from build123d import *

# Parameters (mm, degrees)
SKETCH1_R           = 3.555
SKETCH1_R_2         = 2.5
BOSS_EXTRUDE3_DEPTH = 6.35
BOSS_EXTRUDE4_START = -1.27
SKETCH1_5_R         = 3.555
SKETCH1_5_R_2       = 2.5
BOSS_EXTRUDE4_DEPTH = 1.27


with BuildPart() as part:
    # Sketch1 → Boss-Extrude3 (new body)
    # profile 1 of 2: a face of its own
    with BuildSketch(Plane.XY):
        Polygon((4.725, -2.271873309), (4.725, 2.271873309), (0.79, 4.543746619), (-3.145, 2.271873309), (-3.145, -2.271873309), (0.79, -4.543746619), align=None)
        with Locations((0.79, 0)):
            Circle(SKETCH1_R, mode=Mode.SUBTRACT)
    # profile 2 of 2: a face of its own
    with BuildSketch(Plane.XY):
        with Locations((0.79, 0)):
            Circle(SKETCH1_R)
        Circle(SKETCH1_R_2, mode=Mode.SUBTRACT)
    extrude(amount=BOSS_EXTRUDE3_DEPTH)

    # Sketch1_5 → Boss-Extrude4 (add)
    with BuildSketch(Plane.XY.offset(BOSS_EXTRUDE4_START)):
        with Locations((0.79, 0)):
            Circle(SKETCH1_5_R)
        Circle(SKETCH1_5_R_2, mode=Mode.SUBTRACT)
    extrude(amount=BOSS_EXTRUDE4_DEPTH)


solid = part.part
Here's how the part is built. I have some questions about the finished solid (model axes, mm). A direction names the side the tool comes from. Give positions to 0.01 mm unless a question says otherwise; leave off trailing zeros. Order: outer loops, then holes, each group sorted by start corner. A loop starts at its lowest first (then second) coordinate and runs counter-clockwise, first axis right, second up. Notation, with made-up numbers: M 14,81 L 51,81 A28 cw 51,111 Z; hole C -19,59 d10. An arc over 180 degrees is marked long. Answer as a JSON object with one key per item and string values. Group by question number.
1) Suppose I cut it at C-C, the plane y = 0. Write out the boundary of the cut face in (x, z) (3 decimals), plus the area to 3 significant figures.
2) We'd pull the mould along X, two halves only. Please class faces 3 (the cylindrical face through (-0.54, -2.44, 2.49)), 4 (the flat face through (3, 0, -1.27)), 5 (the cylindrical face through (4.18, 1.07, -0.64)), 6 (the flat face through (4.725, 0, 3)): pulls with the +X half, pulls with the -X half, needs draft (parallel to the pull), parting line crosses it, or undercut.
3) Suppose I cut it at B-B, the plane x = 0. Write out the boundary of the cut face in (y, z).
4) Suppose I cut it at D-D, the plane x = 3. Write out the boundary of the cut face in (y, z), plus the area to 3 significant figures.
5) I'm going to push a flat-ended pin straight in: pin 1 Ø4 at (x, z) = (4, 5) entering from -Y. Where does the tip first touch, or does it pass through?
6) Please list where these lines run through material, in increasing order: L1, parallel to Y at x = -0.75, z = 1; L2, parallel to Z at x = -2.75, y = 1.5; L3, parallel to Y at x = 0, z = 2.75. Write a range as [from, to].
7) Suppose I cut it at A-A, the plane z = 2.5. Write out the boundary of the cut face in (x, y) (3 decimals), plus the area to 3 significant figures.
8) On a 3-axis mill with a long thin cutter (end or side, diameter ignored), from which of +Z, -Z, +X, -X, +Y, -Y can I reach the whole of each face in a straight line? I mean faces 1 (the flat face through (1, -4, 0)), 2 (the flat face through (2.73, -3.424, 3.131)). Say none if no direction works.
Results found:
{
 "1": {"outline": "M -3.145,0 L -2.765,0 L -2.765,-1.27 L -2.5,-1.27 L -2.5,6.35 L -3.145,6.35 Z; M 2.5,-1.27 L 4.345,-1.27 L 4.345,0 L 4.725,0 L 4.725,6.35 L 2.5,6.35 Z", "area": "20.9 mm²"},
 "2": {"face 3": "undercut", "face 4": "needs draft", "face 5": "parting line crosses it", "face 6": "pulls with the +X half"},
 "3": {"outline": "M -4.09,0 L -3.47,0 L -3.47,-1.27 L -2.5,-1.27 L -2.5,6.35 L -4.09,6.35 Z; M 2.5,-1.27 L 3.47,-1.27 L 3.47,0 L 4.09,0 L 4.09,6.35 L 2.5,6.35 Z"},
 "4": {"outline": "M -3.27,0 L -2.78,0 L -2.78,-1.27 L 2.78,-1.27 L 2.78,0 L 3.27,0 L 3.27,6.35 L -3.27,6.35 Z", "area": "48.6 mm²"},
 "5": {"pin 1": "y = -3.85"},
 "6": {"L1": "[-3.65, -2.38], [2.38, 3.65]", "L2": "[0, 6.35]", "L3": "[-4.09, -2.5], [2.5, 4.09]"},
 "7": {"outline": "M -3.145,-2.272 L 0.79,-4.544 L 4.725,-2.272 L 4.725,2.272 L 0.79,4.544 L -3.145,2.272 Z; hole C 0,0 d5", "area": "34.0 mm²"},
 "8": {"face 1": "-Z", "face 2": "+Z, -Z, +X, -Y"}
}
